```python
from build123d import *

# Parameters (mm, degrees)
F0_R     = 4
F1_DEPTH = 100
F2_R     = 3
F3_DEPTH = 2
F4_R     = 4.5
F4_R_2   = 3
F5_DEPTH = 2


with BuildPart() as f1:
    # F0 (on Right) → F1 (new body)
    with BuildSketch(Plane.YZ):
        Circle(F0_R)
    extrude(amount=F1_DEPTH)

    # F2 (on face) → F3 (join)
    with BuildSketch(Plane.YZ.offset(100)):
        Circle(F2_R)
    extrude(amount=F3_DEPTH)

    # F4 (on face) → F5 (join)
    with BuildSketch(Plane.YZ.offset(102)):
        Circle(F4_R)
        Circle(F4_R_2, mode=Mode.SUBTRACT)
        Circle(F4_R_2)
    extrude(amount=F5_DEPTH)

    # F6: F1 across plane


with BuildPart() as f1_1:
    add(f1.part)
    add(f1.part.mirror(Plane.YZ))


solid = f1_1.part
```
Design review of the part built by this model. Coordinates are the model's own, in mm. A direction names the side the tool comes from. Round coordinates to 2 decimals unless told otherwise and drop trailing zeros. Order: outer loops, then holes, each group sorted by start corner. A loop starts at its lowest first (then second) coordinate and runs counter-clockwise, first axis right, second up. Notation, with made-up numbers: (34.5, 36) - (84.5, 36) arc R25 cw to (84.5, 57) - close; hole circle Ø4 at (24, 4.5). An arc over 180 degrees is marked (long way). Return JSON: item names as keys, results as strings.
Q1. For pin 1 Ø3 at (x, z) = (22, -1.5) entering from +Y, flat-tipped, find the tip position at first contact; note if it passes through.
Computed values:
{"pin 1": "stops at y = 4"}
Q2. The part is to be moulded in two halves that separate along X. For faces 3 (the cylindrical face through (102.99, -0.59, 4.46)), 4 (the cylindrical face through (101, -3, 0)), 5 (the flat face through (102, 1, -3)), 6 (the flat face through (104, 0, 0)), say which applies: pulls with the +X half, pulls with the -X half, needs draft (parallel to the pull), parting line crosses it, or undercut.
Computed values:
{"face 3": "needs draft", "face 4": "undercut", "face 5": "undercut", "face 6": "pulls with the +X half"}
Q3. Machinability: for faces 1 (the cylindrical face through (-101, -3, 0)), 2 (the flat face through (-104, 0, 0)), which of the approach directions +Z, -Z, +X, -X, +Y, -Y give a long, thin tool a straight path to every point of the face, cutting with its end or side? Answer none if there is none.
Computed values:
{"face 1": "none", "face 2": "+Z, -Z, -X, +Y, -Y"}
Q4. Consider section A-A on z = 0. Write out the cut boundary in (x, y).
Computed values:
{"outline": "(-104, -4.5) - (-102, -4.5) - (-102, -3) - (-100, -3) - (-100, -4) - (100, -4) - (100, -3) - (102, -3) - (102, -4.5) - (104, -4.5) - (104, 4.5) - (102, 4.5) - (102, 3) - (100, 3) - (100, 4) - (-100, 4) - (-100, 3) - (-102, 3) - (-102, 4.5) - (-104, 4.5) - close"}
Q5. Consider section C-C on x = 87.5. Write out the cut boundary in (y, z).
Computed values:
{"outline": "circle Ø8 at (0, 0)"}
Q6. Wall thickness on L1, parallel to X at y = -3, z = 3.25; L2, parallel to X at y = -1.5, z = 3.5; L3, parallel to Y at x = -48, z = -0.5: over which ranges is each line inside the solid? List them lowest first. Write a range as [from, to].
Computed values:
{"L1": "x = [-104, -102], [102, 104]", "L2": "x = [-104, -102], [-100, 100], [102, 104]", "L3": "y = [-3.97, 3.97]"}
